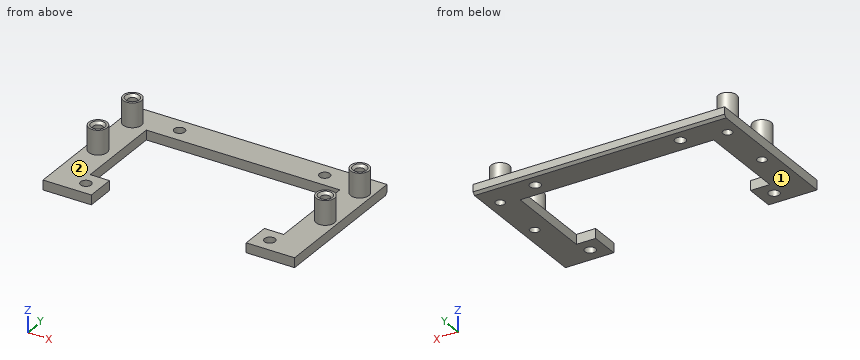
Solid Edge part; units mm, degrees
sketch "Sketch1" plane through (0, 0, 0) normal (0, 0, 1) x (1, 0, 0)
  line L0 (-26, 6) -> (26, 6)
  line L1 (26, 6) -> (26, -24.6)
  line L2 (26, -24.6) -> (20, -24.6)
  line L3 (20, -24.6) -> (20, 0)
  line L4 (20, 0) -> (-20, 0)
  line L5 (-20, 0) -> (-20, -24.6)
  line L6 (-20, -24.6) -> (-26, -24.6)
  line L7 (-26, -24.6) -> (-26, 6)
  dimension "D1" = 26
  dimension "D2" = 20
  dimension "D3" = 26
extrude "Protrusion1" add sketch "Sketch1" along normal blind 2
sketch "Sketch2" plane through (0, -11, 2) normal (0, 0, 1) x (1, 0, 0)
  circle A0 centre (15, 14) radius 1.1
  circle A1 centre (-15, 14) radius 1.1
  dimension "D1" = 15
extrude "Cutout1" cut sketch "Sketch2" against normal through all
chamfer "Chamfer1" distance 0.5 angle 45 1 edges at (0, 6, 0)
sketch "Sketch3" plane through (0, -11, 2) normal (0, 0, 1) x (0, -1, 0)
  circle A0 centre (-12, 23.5) radius 1.9
  circle A1 centre (-0.6, 23.5) radius 1.9
  circle A2 centre (-0.6, -23.5) radius 1.9
  circle A3 centre (-12, -23.5) radius 1.9
  dimension "D1" = 12
extrude "Extrusionsausprägung_2" add sketch "Sketch3" along normal blind 5
sketch "Sketch4" plane through (23.5, 1, 7) normal (0, 0, 1) x (0, -1, 0)
  circle A0 centre (0, 0) radius 0.95
  circle A1 centre (11.4, 0) radius 0.95
  circle A2 centre (0, -47) radius 0.95
  circle A3 centre (11.4, -47) radius 0.95
extrude "Cutout2" cut sketch "Sketch4" against normal through all
chamfer "Fase_2" distance 0.5 angle 45 4 edges at (23.5, 1.95, 7) (23.5, -9.45, 7) (-23.5, 1.95, 7) (-23.5, -9.45, 7)
sketch "Sketch5" plane through (0, -9.3, 2) normal (0, 0, 1) x (0, -1, 0)
  line L0 (9.3, -16) -> (15.3, -16)
  line L1 (15.3, -16) -> (15.3, -26)
  line L2 (15.3, -26) -> (3.3, -26)
  line L3 (3.3, -26) -> (3.3, -20)
  line L4 (3.3, -20) -> (9.3, -20)
  line L5 (9.3, -20) -> (9.3, -16)
  line L6 (9.3, 16) -> (15.3, 16)
  line L7 (15.3, 16) -> (15.3, 26)
  line L8 (15.3, 26) -> (3.3, 26)
  line L9 (3.3, 26) -> (3.3, 20)
  line L10 (3.3, 20) -> (9.3, 20)
  line L11 (9.3, 20) -> (9.3, 16)
  dimension "D1" = 15.3
  dimension "D2" = 9.3
  dimension "D3" = 15.3
  dimension "D4" = 15.3
  dimension "D5" = 15.3
extrude "Extrusionsausprägung_3" add sketch "Sketch5" against normal blind 2
sketch "Sketch6" plane through (0, -9.3, 2) normal (0, 0, 1) x (0, -1, 0)
  circle A0 centre (12.3, 19) radius 1.1
  circle A1 centre (12.3, -19) radius 1.1
  dimension "D1" = 12.3
  dimension "D2" = 12.3
extrude "Cutout3" cut sketch "Sketch6" against normal through all
CAD build for the part. Positions are in the model's coordinates, mm. Face numbers are marked on the shaded views. Give positions to 0.01 mm unless a question says otherwise; leave off trailing zeros. Order: outer loops, then holes, each group sorted by start corner. A loop starts at its lowest first (then second) coordinate and runs counter-clockwise, first axis right, second up. Notation, with made-up numbers: (29.25, 6.5) -> (82.25, 6.5) arc R10 cw to (82.25, 17.5) -> close; hole circle Ø11 at (-26, 70.25). An arc over 180 degrees is marked (long way). Return JSON: item names as keys, results as strings.
Q1. Drill centre lines: line 1 (Z direction, x = 23.5, y = -13); line 2 (X direction, y = -0.5, z = 6.5). Where is each one in solid material? Low to high.
Working result:
{"line 1": "0 to 2", "line 2": "-24.67 to -22.33, 22.33 to 24.67"}
Q2. Saw through at D-D (x = 15). Write the cut outline in (y, z), then the cut area to 4 significant figures.
Working result:
{"outline": "(0, 0) -> (1.9, 0) -> (1.9, 2) -> (0, 2) -> close; (4.1, 0) -> (5.5, 0) -> (6, 0.5) -> (6, 2) -> (4.1, 2) -> close", "area": "7.475 mm²"}
Q3. Saw through at B-B (x = -19). Write the cut outline in (y, z), then the cut area to 3 significant figures.
Working result:
{"outline": "(-24.6, 0) -> (-22.7, 0) -> (-22.7, 2) -> (-24.6, 2) -> close; (-20.5, 0) -> (-18.6, 0) -> (-18.6, 2) -> (-20.5, 2) -> close; (0, 0) -> (5.5, 0) -> (6, 0.5) -> (6, 2) -> (0, 2) -> close", "area": "19.5 mm²"}
Q4. Flat gauge pins, fed straight in: pin 1 (3 mm diameter, centred on x = 23.5, y = 1, fed in from -Z); pin 2 (2 mm diameter, centred on y = 1, z = 3.5, fed in from +X); pin 3 (3 mm diameter, centred on x = 15, y = 3, fed in from +Z); pin 4 (1.6 mm diameter, centred on x = 4, z = 0.5, fed in from -Y). Where does each tip first touch, or does it go through?
Working result:
{"pin 1": "z = 0", "pin 2": "x = 25.4", "pin 3": "z = 2", "pin 4": "y = 0"}
Q5. Saw through at A-A (z = 5.25). Write the cut outline in (x, y).
Working result:
{"outline": "circle Ø3.8 at (-23.5, -10.4); circle Ø3.8 at (-23.5, 1); circle Ø3.8 at (23.5, -10.4); circle Ø3.8 at (23.5, 1); hole circle Ø1.9 at (-23.5, -10.4); hole circle Ø1.9 at (-23.5, 1); hole circle Ø1.9 at (23.5, -10.4); hole circle Ø1.9 at (23.5, 1)"}
Q6. Saw through at C-C (y = -17.5). Write the cut outline in (x, z).
Working result:
{"outline": "(-26, 0) -> (-20, 0) -> (-20, 2) -> (-26, 2) -> close; (20, 0) -> (26, 0) -> (26, 2) -> (20, 2) -> close"}
Q7. Mould opens along X. For the marked faces 1 and 2 say: pulls with the +X half, pulls with the -X half, needs draft (parallel to the pull), parting line crosses it, or undercut.
Working result:
{"face 1": "needs draft", "face 2": "undercut"}
